from build123d import *

# Parameters (mm, degrees)
F0_W     = 23.9999974624
F0_H     = 73.9999974624
F1_DEPTH = 25
F0_W_2   = 20
F0_H_2   = 6.8478258327
F2_DEPTH = 2.5
F3_SIZE  = 0.99999


# Not quite as in the source:
# - a fillet or chamfer is up to 0.001 mm smaller than in the source, because OpenCascade refuses the exact size


with BuildPart() as f1:
    # F0 (on Top) → F1 (new body)
    with BuildSketch(Plane.XY):
        with Locations((-2.6413043961, 7.5985620491)):
            Rectangle(F0_W, F0_H)
        Polygon((-12.6413043961, 12.7173913643), (-12.6413043961, 42.5985620491), (7.3586956039, 42.5985620491), (7.3586956039, 12.7173913643), (7.3586956039, 5.8695655316), (7.3586956039, -27.4014379509), (-12.6413043961, -27.4014379509), (-12.6413043961, 5.8695655316), align=None, mode=Mode.SUBTRACT)
    extrude(amount=F1_DEPTH)

    # F0 (on Top) → F2 (join)
    with BuildSketch(Plane.XY):
        with Locations((-2.6413043961, 7.5985620491)):
            Rectangle(F0_W, F0_H)
        Polygon((-12.6413043961, 12.7173913643), (-12.6413043961, 42.5985620491), (7.3586956039, 42.5985620491), (7.3586956039, 12.7173913643), (7.3586956039, 5.8695655316), (7.3586956039, -27.4014379509), (-12.6413043961, -27.4014379509), (-12.6413043961, 5.8695655316), align=None, mode=Mode.SUBTRACT)
        with Locations((-2.6413043961, 9.2934784479)):
            Rectangle(F0_W_2, F0_H_2)
    extrude(amount=F2_DEPTH)

    # F3 (size 1 in the source; OpenCascade refuses exactly that, so slightly less here)
    f3_edges = [f1.edges().sort_by_distance(p)[0] for p in [
        (-2.641304, -29.401437, 25),
        (-14.641303, 7.598562, 25),
        (9.358694, 7.598562, 25),
        (-2.641304, 44.598561, 25),
        (-2.641304, 42.598562, 25),
        (7.358696, 7.598562, 25),
        (-12.641304, 7.598562, 25),
        (-2.641304, -27.401438, 25),
    ]]
    chamfer(f3_edges, length=F3_SIZE)


solid = f1.part
Part model, mm, in its own coordinate system. A direction names the side the tool comes from. Coordinates: 2 decimals unless noted, no trailing zeros. Order: outer loops, then holes, each group sorted by start corner. A loop starts at its lowest first (then second) coordinate and runs counter-clockwise, first axis right, second up. Notation, with made-up numbers: M -37,80.5 L -12,80.5 A17 ccw -12,105.5 Z; hole C -24,1 d10. An arc over 180 degrees is marked long. Use a Markdown table: item, result.
(1) Pull direction X, two halves, no side cores. Call faces 3 (the flat face through (-3, 44.599, 12)), 4 (the flat face through (9.359, 7, 12)), 5 (the flat face through (-3, 9, 2.5)): released by +X, released by -X, zero draft, split by the parting line, or undercut.
A:
| item | result |
|---|---|
| face 3 | zero draft |
| face 4 | released by +X |
| face 5 | undercut |
(2) Tool access for faces 1 (the flat face through (-4, 8, 0)), 2 (the flat face through (-3, 12.717, 1)): list every direction of +Z, -Z, +X, -X, +Y, -Y with a clear straight run to the whole face (end or side of a thin tool).
A:
| item | result |
|---|---|
| face 1 | -Z, +X, -X, +Y, -Y |
| face 2 | +Z, -Z |
(3) Cut at A-A on x = 3.5. State how many separate pieces and enclosed holes the cut face has, then the cut area to 3 significant figures.
A:
| item | result |
|---|---|
| separate pieces | 3 |
| enclosed holes | 0 |
| area | 115 mm^2 |
(4) Cut at C-C on z = 13. Write the cut outline in (x, y).
A:
| item | result |
|---|---|
| outline | M -14.64,-29.4 L 9.36,-29.4 L 9.36,44.6 L -14.64,44.6 Z; hole M -12.64,-27.4 L 7.36,-27.4 L 7.36,42.6 L -12.64,42.6 Z |
(5) Flat gauge pins, fed straight in: pin 1 (10 mm diameter, centred on x = 3, y = -7, fed in from +Z); pin 2 (5.5 mm diameter, centred on x = 0, y = 10, fed in from +Z). Where does each tip first touch, or does it go through?
A:
| item | result |
|---|---|
| pin 1 | stops at z = 24.64 |
| pin 2 | stops at z = 2.5 |
(6) Probe L1, parallel to Y at x = 7.25, z = 16.5; L2, parallel to X at y = 25, z = 8.75; L3, parallel to Z at x = 5.75, y = 9. List the from-to ranges inside material, lowest first.
A:
| item | result |
|---|---|
| L1 | y = -29.4 to -27.4, 42.6 to 44.6 |
| L2 | x = -14.64 to -12.64, 7.36 to 9.36 |
| L3 | z = 0 to 2.5 |
